```python
from build123d import *

# Parameters (mm, degrees)
F0_W     = 254
F0_H     = 12.7
F1_DEPTH = 127
F2_W     = 12.7
F2_H     = 114.3
F3_DEPTH = 127
F4_W     = 12.7
F4_H     = 114.3
F5_DEPTH = 127


with BuildPart() as f1:
    # F0 (on Top) → F1 (new body)
    with BuildSketch(Plane.XY):
        with Locations((-22.784118, 50.164945)):
            Rectangle(F0_W, F0_H)
    extrude(amount=F1_DEPTH)

    # F2 (on Top) → F3 (join)
    with BuildSketch(Plane.XY):
        with Locations((-143.434073, -13.334987)):
            Rectangle(F2_W, F2_H)
    extrude(amount=F3_DEPTH)

    # F4 (on Top) → F5 (join)
    with BuildSketch(Plane.XY):
        with Locations((97.865868, -13.334994)):
            Rectangle(F4_W, F4_H)
    extrude(amount=F5_DEPTH)


solid = f1.part
```
Design review of the part built by this model. Coordinates are the model's own, in mm. A direction names the side the tool comes from. Coordinates: 2 decimals unless noted, no trailing zeros. Write each loop counter-clockwise with the first axis right and the second up, starting at its lowest first coordinate (ties: lowest second). Pieces come first, ordered by that corner, then holes. Notation, with made-up numbers: M 0.25,-12 L 54.25,-12 A20 ccw 54.25,0 Z; hole C -16.5,81.5 d10. An arc over 180 degrees is marked long. Answer as a JSON object with one key per item and string values.
Item 1: Wall thickness on probe 1 along X at (y, z) = (4, 97); probe 2 along Y at (x, z) = (-5, 53): over which ranges is each line inside the solid? List them lowest first.
Outcome:
{"probe 1": "-149.78 to -137.08, 91.52 to 104.22", "probe 2": "43.81 to 56.51"}
Item 2: Draft analysis for pull direction X (two halves, no side actions). For faces 1 (the flat face through (-24, 43.815, 63)), 2 (the flat face through (-23, 45, 127)), 3 (the flat face through (104.216, 50, 63)), state which applies: pulls with the +X half, pulls with the -X half, needs draft (parallel to the pull), parting line crosses it, or undercut.
Outcome:
{"face 1": "undercut", "face 2": "needs draft", "face 3": "pulls with the +X half"}
Item 3: Add section C-C, the plane x = 4.5. Give the boundary of the cut face in (y, z).
Outcome:
{"outline": "M 43.81,0 L 56.51,0 L 56.51,127 L 43.81,127 Z"}
Item 4: Insertion check: pin 1 Ø3 at (x, z) = (-2, 37) entering from -Y. The pin has a flat end and moves straight along its axis. Give the tip position at first contact, or say it passes through.
Outcome:
{"pin 1": "y = 43.81"}
Item 5: Machinability: for faces 4 (the flat face through (91.516, -14, 63)), 5 (the flat face through (-149.784, -14, 63)), which of the approach directions +Z, -Z, +X, -X, +Y, -Y give a long, thin tool a straight path to every point of the face, cutting with its end or side? Answer none if there is none.
Outcome:
{"face 4": "+Z, -Z, -Y", "face 5": "+Z, -Z, -X, +Y, -Y"}
Item 6: Add section A-A, the plane y = -14.5. Give the boundary of the cut face in (x, z), and give its area (3 significant figures).
Outcome:
{"outline": "M -149.78,0 L -137.08,0 L -137.08,127 L -149.78,127 Z; M 91.52,0 L 104.22,0 L 104.22,127 L 91.52,127 Z", "area": "3,230 mm²"}
